```python
from build123d import *

# Parameters (mm, degrees)
SKETCH1_W           = 203.2
SKETCH1_H           = 203.2
BOSS_EXTRUDE1_DEPTH = 3.175
CUT_EXTRUDE1_DEPTH  = 6.35
SKETCH3_R           = 4.953
SKETCH3_R_2         = 13.335
CUT_EXTRUDE2_DEPTH  = 12.7
CUT_EXTRUDE3_START  = -3.175
SKETCH4_R           = 84.1375
SKETCH4_R_2         = 76.2
CUT_EXTRUDE3_DEPTH  = 3.175


with BuildPart() as part:
    # Sketch1 → Boss-Extrude1 (new, symmetric)
    with BuildSketch(Plane(origin=(0, 0, 0), x_dir=(1, 0, 0), z_dir=(0, 1, 0))):
        Rectangle(SKETCH1_W, SKETCH1_H)
    extrude(amount=BOSS_EXTRUDE1_DEPTH, both=True)

    # Sketch2 → Cut-Extrude1 (cut, symmetric)
    with BuildSketch(Plane(origin=(0, 0, 0), x_dir=(1, 0, 0), z_dir=(0, 1, 0))):
        with BuildLine():
            Line((53.975, -64.543150537), (53.975, 64.543150537))
            ThreePointArc((53.975, 64.543150537), (84.1375, 0), (53.975, -64.543150537))
        make_face()
    extrude(amount=CUT_EXTRUDE1_DEPTH, both=True, mode=Mode.SUBTRACT)

    # Sketch3 → Cut-Extrude2 (cut)
    with BuildSketch(Plane(origin=(0, 3.175, 0), x_dir=(1, 0, 0), z_dir=(0, 1, 0))):
        with Locations(Location((-34.925, -34.925, 0), (0, 0, 270))):
            Circle(SKETCH3_R)
        with Locations(Location((-34.925, 34.925, 0), (0, 0, 270))):
            Circle(SKETCH3_R)
        with Locations(Location((34.925, 34.925, 0), (0, 0, 270))):
            Circle(SKETCH3_R)
        with Locations(Location((34.925, -34.925, 0), (0, 0, 270))):
            Circle(SKETCH3_R)
        with Locations(Location((0, 0, 0), (0, 0, 270))):
            Circle(SKETCH3_R_2)
    extrude(amount=-CUT_EXTRUDE2_DEPTH, mode=Mode.SUBTRACT)

    # Sketch4 → Cut-Extrude3 (cut)
    with BuildSketch(Plane.XZ.offset(3.175).offset(CUT_EXTRUDE3_START)):
        with Locations(Location((0, 0, 0), (0, 0, 50.095533509))):
            Circle(SKETCH4_R)
        Circle(SKETCH4_R_2, mode=Mode.SUBTRACT)
    extrude(amount=CUT_EXTRUDE3_DEPTH, mode=Mode.SUBTRACT)


solid = part.part
```
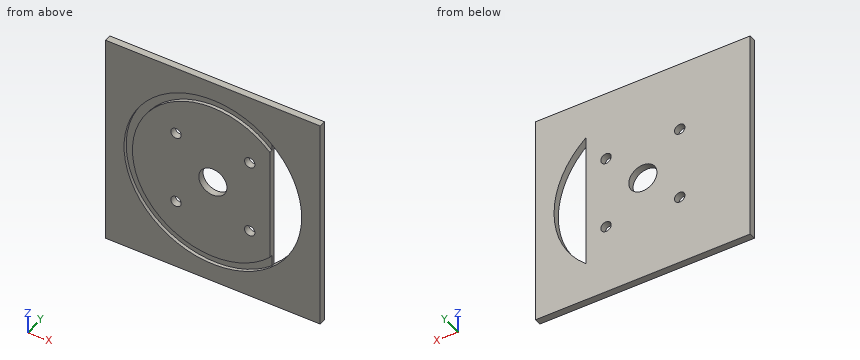
The listing builds one solid part. Answer for the finished solid, in the listing's coordinates (mm). Coordinates: 2 decimals unless noted, no trailing zeros. Loops run counter-clockwise (first coordinate to the right, second up) from the corner with the lowest first, then second, coordinate; pieces in that order, holes last. Notation, with made-up numbers: (22, -22) -> (32, -22) arc R31 cw to (32, 9) -> close; hole circle Ø5 at (67.5, -5.5). An arc over 180 degrees is marked (long way). Use one line per item in the form item = value. Start each with the question number.
Item 1: The part is cut by section A-A on z = 0. Determine the outline of the cut face in (x, y) (1 decimal).
Item 2: The part is cut by section C-C on x = 66.5. Determine the outline of the cut face in (y, z) (3 decimals), then the cut area to 3 significant figures.
Item 3: Consider L1, parallel to X at y = -1, z = 1 (3 decimals); L2, parallel to X at y = -2.5, z = -22.5 (3 decimals); L3, parallel to Z at x = -49, y = -2.5. Determine where each line is inside the solid, lowest interval first. Write a range as [from, to].
Item 4: The part is cut by section B-B on x = 0. Determine the outline of the cut face in (y, z) (1 decimal).
Answer key:
q1.outline = (-101.6, -3.2) -> (-84.1, -3.2) -> (-84.1, 0) -> (-76.2, 0) -> (-76.2, -3.2) -> (-13.3, -3.2) -> (-13.3, 3.2) -> (-101.6, 3.2) -> close; (13.3, -3.2) -> (54, -3.2) -> (54, 3.2) -> (13.3, 3.2) -> close; (84.1, -3.2) -> (101.6, -3.2) -> (101.6, 3.2) -> (84.1, 3.2) -> close
q2.outline = (-3.175, -101.6) -> (3.175, -101.6) -> (3.175, -51.545) -> (-3.175, -51.545) -> close; (-3.175, 51.545) -> (3.175, 51.545) -> (3.175, 101.6) -> (-3.175, 101.6) -> close
q2.area = 636 mm2
q3.L1 = [-101.6, -84.132], [-76.193, -13.297], [13.297, 53.975], [84.132, 101.6]
q3.L2 = [-101.6, -81.073], [-72.802, 53.975], [81.073, 101.6]
q3.L3 = [-101.6, -68.4], [-58.36, 58.36], [68.4, 101.6]
q4.outline = (-3.2, -101.6) -> (3.2, -101.6) -> (3.2, -13.3) -> (-3.2, -13.3) -> (-3.2, -76.2) -> (0, -76.2) -> (0, -84.1) -> (-3.2, -84.1) -> close; (-3.2, 13.3) -> (3.2, 13.3) -> (3.2, 101.6) -> (-3.2, 101.6) -> (-3.2, 84.1) -> (0, 84.1) -> (0, 76.2) -> (-3.2, 76.2) -> close
